Autodesk Inventor part; units mm, degrees
ref_plane "YZ Plane" through (0, 0, 0) normal (1, 0, 0) x (0, 1, 0)
ref_plane "XZ Plane" through (0, 0, 0) normal (0, 1, 0) x (-1, 0, 0)
ref_plane "XY Plane" through (0, 0, 0) normal (0, 0, 1) x (1, 0, 0)
sketch "Sketch1" plane through (0, 0, 0) normal (0, 0, 1) x (1, 0, 0)
  circle A0 centre (0, 0) radius 6.25
  dimension "d0" = 12.5
extrude "Extrusion1" add sketch "Sketch1" along normal blind 1.5
sketch "axles" plane through (0, 0, 0) normal (0, 0, 1) x (1, 0, 0)
  point P0 (0, 0)
  point P1 (7, 0)
  point P2 (0.3, 0)
  dimension "d3" = 7
  dimension "d4" = 6.7
sketch "Sketch4" plane through (0, 0, 1.5) normal (0, 0, 1) x (1, 0, 0)
  circle A0 centre (0, 0) radius 2.65
  dimension "d8" = 5.3
extrude "Extrusion3" add sketch "Sketch4" along normal blind 4.2
chamfer "Chamfer1" distance 0.8 angle 45 1 edges at (-2.65, 0, 5.7)
sketch "Sketch5" plane through (0, 0, 0) normal (0, 0, 1) x (1, 0, 0)
  circle A0 centre (0.3, 0) radius 1.6
  point P0 (0, 0)
  dimension "d14" = 3.2
extrude "motor shaft" cut sketch "Sketch5" along normal blind 2.5
sketch "Sketch6" plane through (0, 0, 0) normal (0, 0, -1) x (-1, 0, 0)
  circle A0 centre (-7, 0) radius 6.25
  point P0 (0, 0)
  dimension "d17" = 12.5
extrude "Extrusion5" cut sketch "Sketch6" against normal blind 2.5
sketch "Sketch8" plane through (0, 0, 5.7) normal (0, 0, 1) x (1, 0, 0)
  point P0 (0, 0)
  point P1 (0, 0)
hole "Hole1" at (0, 0, 5.7) direction (0, 0, -1) diameter 1.2 end through all
fillet "Fillet1" radius 1 2 edges at (3.5, 5.1781, 0.75) (3.5, -5.1781, 0.75)
sketch "Sketch9" plane through (0, 0, 1.5) normal (0, 0, 1) x (1, 0, 0)
  line L0 (0, -4.25) -> (0, 4.25) construction
  point P0 (0, 0)
  point P1 (0, 0)
  dimension "d28" = 8.5
hole "Hole2" at (0, -4.25, 1.5) at (0, 4.25, 1.5) direction (0, 0, -1) diameter 1.5 end through all counterbore diameter 2.5 counterbore depth 1.1
equation "\"axle_dist_2_3__3_4\" = 7"
equation "\"axle_dist_1_2\" = 6.7"
properties part number "gearbox_axle3_support"
The model under review builds one solid part; all positions refer to its coordinate system, in mm. A direction names the side the tool comes from. Round coordinates to 2 decimals unless told otherwise and drop trailing zeros. Write each loop counter-clockwise with the first axis right and the second up, starting at its lowest first coordinate (ties: lowest second). Pieces come first, ordered by that corner, then holes. Notation, with made-up numbers: (75.5, 19.5) - (94.5, 19.5) arc R11 cw to (94.5, 30.5) - close; hole circle Ø8 at (21.5, 20). An arc over 180 degrees is marked (long way). One line per item, written item: value. Start each with the question number.
1. Consider section B-B on z = 4.2. Write out the cut boundary in (x, y), and give its area (3 significant figures).
2. The part is to be moulded in two halves that separate along Y. For faces 1 (the face through (1.33, 2.63, 0.95)), 2 (the face through (-6.248, -0.167, 0.74)), 3 (the face through (-3, 0, 1.5)), say which applies: released by +Y, released by -Y, zero draft, split by the parting line, or undercut.
3. Consider section A-A on y = 0. Write out the cut boundary in (x, z), and give its area (3 significant figures).
4. To check wall thickness, follow L1, parallel to Y at x = 0.3, z = 1.4; L2, parallel to Z at x = 1.25, y = -0.75; L3, parallel to Z at x = -4, y = 2. State the ranges of each line that lie inside material, in increasing order. Write a range as from..to.
5. Clearance check with flat-ended pins moving along their axes: P1, Ø2, axis at x = 0, y = -4.25, coming from the +Z side; P2, Ø1, axis at x = -1.5, y = -2, coming from the +Z side; P3, Ø3, axis at x = 0, y = -4, coming from the +Z side; P4, Ø0.8, axis at x = 0, y = 4.5, coming from the +Z side. State where each tip first meets the part, or that it passes through.
6. Machinability: for faces 4 (the face through (-1.3, 0, 1.2)), 5 (the face through (1.35, -2.67, 0.95)), 6 (the face through (-2.647, -0.117, 3.554)), which of the approach directions +Z, -Z, +X, -X, +Y, -Y give a long, thin tool a straight path to every point of the face, cutting with its end or side? Answer none if there is none.
7. Consider section D-D on y = -3.75. Write out the cut boundary in (x, z).
8. Consider section C-C on x = 0. State how many separate pieces and enclosed holes the cut face has, and give its area (3 significant figures).
Checks:
1. outline: circle Ø5.3 at (0, 0); hole circle Ø1.2 at (0, 0)
1. area: 20.9 mm^2
2. face 1: undercut
2. face 2: split by the parting line
2. face 3: zero draft
3. outline: (-6.25, 0) - (-1.3, 0) - (-1.3, 2.5) - (-0.6, 2.5) - (-0.6, 5.7) - (-1.85, 5.7) - (-2.65, 4.9) - (-2.65, 1.5) - (-6.25, 1.5) - close; (0.6, 2.5) - (2.65, 2.5) - (2.65, 4.9) - (1.85, 5.7) - (0.6, 5.7) - close
3. area: 21.3 mm^2
4. L1: y = -6.24..-5.46, -3.04..-1.6, 1.6..3.04, 5.46..6.24
4. L2: z = 2.5..5.7
4. L3: z = 0..1.5
5. P1: stops at z = 0.4
5. P2: stops at z = 5.55
5. P3: stops at z = 5.05
5. P4: passes through
6. face 4: -Z
6. face 5: -Z, +X
6. face 6: +Z
7. outline: (-5, 0) - (-0.56, 0) - (-0.56, 0.4) - (-1.15, 0.4) - (-1.15, 1.5) - (-5, 1.5) - close; (0.56, 0) - (2, 0) - (2, 1.5) - (1.15, 1.5) - (1.15, 0.4) - (0.56, 0.4) - close
8. separate pieces: 4
8. enclosed holes: 0
8. area: 22.0 mm^2
